Can you work these out from the model? Positions are in its coordinate system, mm. Face numbers are marked on the shaded views. A direction names the side the tool comes from. Give positions to 0.01 mm unless a question says otherwise; leave off trailing zeros. Loops run counter-clockwise (first coordinate to the right, second up) from the corner with the lowest first, then second, coordinate; pieces in that order, holes last. Notation, with made-up numbers: (30, 24) - (45, 24) arc R14 ccw to (45, 39) - close; hole circle Ø6 at (63.25, -11.75). An arc over 180 degrees is marked (long way). Answer as a JSON object with one key per item and string values.
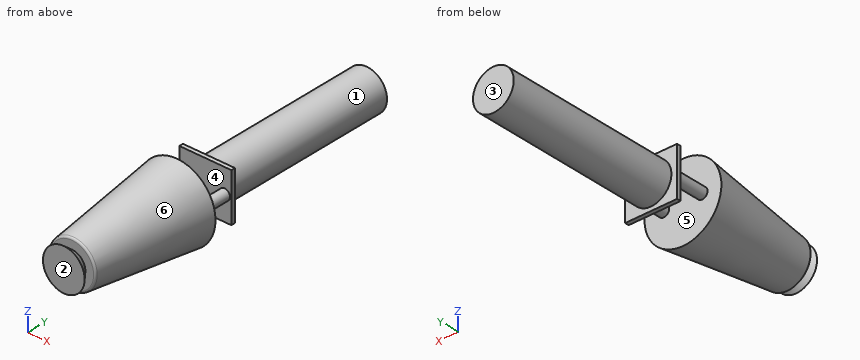
```python
from build123d import *

# Parameters (mm, degrees)
FILLET3_R           = 1
SKETCH2_W           = 2.6733627
SKETCH2_H           = 15.8
SKETCH4_W           = 25.690547406
SKETCH4_H           = 23.95860039
BOSS_EXTRUDE1_DEPTH = 2
SKETCH5_W           = 10.057084603
SKETCH5_H           = 88


with BuildPart() as part:
    # Sketch1 → Revolve1 (revolve)
    with BuildSketch(Plane.XY):
        Polygon((0, 0), (0, 63.2), (19, 63.2), (11.588395286, 4.555292852), (6.627531845, 4.555292852), (10.308172463, 0), align=None)
    revolve(axis=Axis((0, 0, 0), (0, 1, 0)))

    # Fillet3
    fillet3_edges = [part.edges().sort_by_distance(p)[0] for p in [
        (-11.588395286, 4.555292852, 0),
    ]]
    fillet(fillet3_edges, radius=FILLET3_R)

    # Sketch2 → Revolve2 (revolve)
    with BuildSketch(Plane.XY):
        with Locations((10.825435474, 71.1)):
            Rectangle(SKETCH2_W, SKETCH2_H)
    revolve2 = revolve(axis=Axis((9.488754124, 63.2, 0), (0, 1, 0)))

    # Mirror1: Revolve2 across plane
    add(revolve2.mirror(Plane(origin=(0, 0, 0), x_dir=(0, 0, 1), z_dir=(1, 0, 0))))

    # Sketch4 → Boss-Extrude1 (add)
    with BuildSketch(Plane(origin=(0, 79, 0), x_dir=(1, 0, 0), z_dir=(0, 1, 0))):
        Rectangle(SKETCH4_W, SKETCH4_H)
    extrude(amount=BOSS_EXTRUDE1_DEPTH)

    # Sketch5 → Revolve4 (revolve)
    with BuildSketch(Plane.XY):
        with Locations((5.028542301, 125)):
            Rectangle(SKETCH5_W, SKETCH5_H)
    revolve(axis=Axis((0, 81, 0), (0, 1, 0)))


solid = part.part
```
1) Imagine slicing it at C-C on z = 0. Write out the boundary of the cut face in (x, y), and give its area (3 significant figures).
Check sheet entries:
{"outline": "(-19, 63.2) - (-11.7, 5.43) arc R1 ccw to (-10.71, 4.56) - (-6.63, 4.56) - (-10.31, 0) - (10.31, 0) - (6.63, 4.56) - (10.71, 4.56) arc R1 ccw to (11.7, 5.43) - (19, 63.2) - (12.16, 63.2) - (12.16, 79) - (12.85, 79) - (12.85, 81) - (10.06, 81) - (10.06, 169) - (-10.06, 169) - (-10.06, 81) - (-12.85, 81) - (-12.85, 79) - (-12.16, 79) - (-12.16, 63.2) - close; hole (-6.82, 63.2) - (6.82, 63.2) - (6.82, 79) - (-6.82, 79) - close", "area": "3,860 mm2"}
2) Which directions (+Z, -Z, +X, -X, +Y, -Y) give clear straight access to the entire face, cutting with the end or side of a thin tool? Please do the marked faces 1 and 2.
Check sheet entries:
{"face 1": "+Y", "face 2": "+Z, -Z, +X, -X, -Y"}
3) I'm going to push flat-ended pins straight in: P1, Ø3, axis at y = 101, z = -2, coming from the -X side; P2, Ø3, axis at x = 13, z = 4.5, coming from the +Y side; P3, Ø10, axis at y = 123.5, z = 0, coming from the +X side. Where does each tip first touch, or does it pass through?
Check sheet entries:
{"P1": "x = -10.04", "P2": "y = 81", "P3": "x = 10.06"}
4) If we mould it in two halves opening along Y, with no side actions, what happens to the marked faces 3, 4, 5 and 6? For each: released by +Y, released by -Y, zero draft, split by the parting line, or undercut.
Check sheet entries:
{"face 3": "released by +Y", "face 4": "undercut", "face 5": "undercut", "face 6": "released by -Y"}
5) Imagine slicing it at A-A on y = 74. Write out the boundary of the cut face in (x, z), and give its area (3 significant figures).
Check sheet entries:
{"outline": "circle Ø5.35 at (-9.49, 0); circle Ø5.35 at (9.49, 0)", "area": "44.9 mm2"}
6) Imagine slicing it at B-B on x = 0. Write out the boundary of the cut face in (y, z), and give its area (3 significant figures).
Check sheet entries:
{"outline": "(0, -10.31) - (4.56, -6.63) - (4.56, -10.71) arc R1 ccw to (5.43, -11.7) - (63.2, -19) - (63.2, 19) - (5.43, 11.7) arc R1 ccw to (4.56, 10.71) - (4.56, 6.63) - (0, 10.31) - close; (79, -11.98) - (81, -11.98) - (81, -10.06) - (169, -10.06) - (169, 10.06) - (81, 10.06) - (81, 11.98) - (79, 11.98) - close", "area": "3,690 mm2"}
7) Imagine slicing it at D-D on y = 104. Write out the boundary of the cut face in (x, z), and give its area (3 significant figures).
Check sheet entries:
{"outline": "circle Ø20.11 at (0, 0)", "area": "318 mm2"}
8) I need wall thicknesses on L1, parallel to Y at x = -4, z = -6.5; L2, parallel to Y at x = -8, z = -7; L3, parallel to Y at x = 7, z = -6. Which ranges of each line are inside material? Lowest first, please.
Check sheet entries:
{"L1": "0 to 3.31, 4.56 to 63.2, 79 to 169", "L2": "4.56 to 63.2, 79 to 81", "L3": "0 to 1.35, 4.56 to 63.2, 79 to 169"}
